The drawing under review shows one solid part. Ordinate dimensions are in mm from its lowest x, y, z. A direction names the side the tool comes from. Round coordinates to 2 decimals unless told otherwise and drop trailing zeros. Order: outer loops, then holes, each group sorted by start corner. A loop starts at its lowest first (then second) coordinate and runs counter-clockwise, first axis right, second up. Notation, with made-up numbers: (55.5, 55) -> (81.5, 55) arc R17 cw to (81.5, 71) -> close; hole circle Ø2 at (-36, 44). An arc over 180 degrees is marked (long way). Use a Markdown table: item, result. Add a question column.
1) Consider section B-B (y = 10). State the section outline as (x, z) points.
2) Wall thickness on line 1 along Y through (x, z) = (10, 23.85); line 2 along Y through (x, z) = (15.4, 10); line 3 along X through (y, z) = (13.5, 12.25): over which ranges is each line inside the solid? List them lowest first. Write a range as [from, to].
3) Clearance check with flat-ended pins moving along their axes: P1, Ø1.2, axis at x = 10, y = 5, coming from the -Z side; P2, Ø5, axis at x = 12.5, z = 6, coming from the -Y side; P3, Ø5, axis at x = 16, y = 17, coming from the -Z side; P4, Ø2.5, axis at x = 10.5, y = 6, coming from the -Z side. State where each tip first meets the part, or that it passes through.
4) Consider section C-C (z = 22). State the section outline as (x, y) points, plus the area to 3 significant figures.
5) Machinability: for the marked faces 4, 5 and 6, which of the approach directions +Z, -Z, +X, -X, +Y, -Y give a long, thin tool a straight path to every point of the face, cutting with its end or side? Answer none if there is none.
6) Draft analysis for pull direction X (two halves, no side actions). For the marked faces 1, 2 and 3, state which applies: pulls with the +X half, pulls with the -X half, needs draft (parallel to the pull), parting line crosses it, or undercut.
7) Consider section A-A (z = 17.75). State the section outline as (x, y) points, plus the area to 3 significant figures.
8) Consider section D-D (x = 10). State the section outline as (y, z) points, plus the area to 3 significant figures.
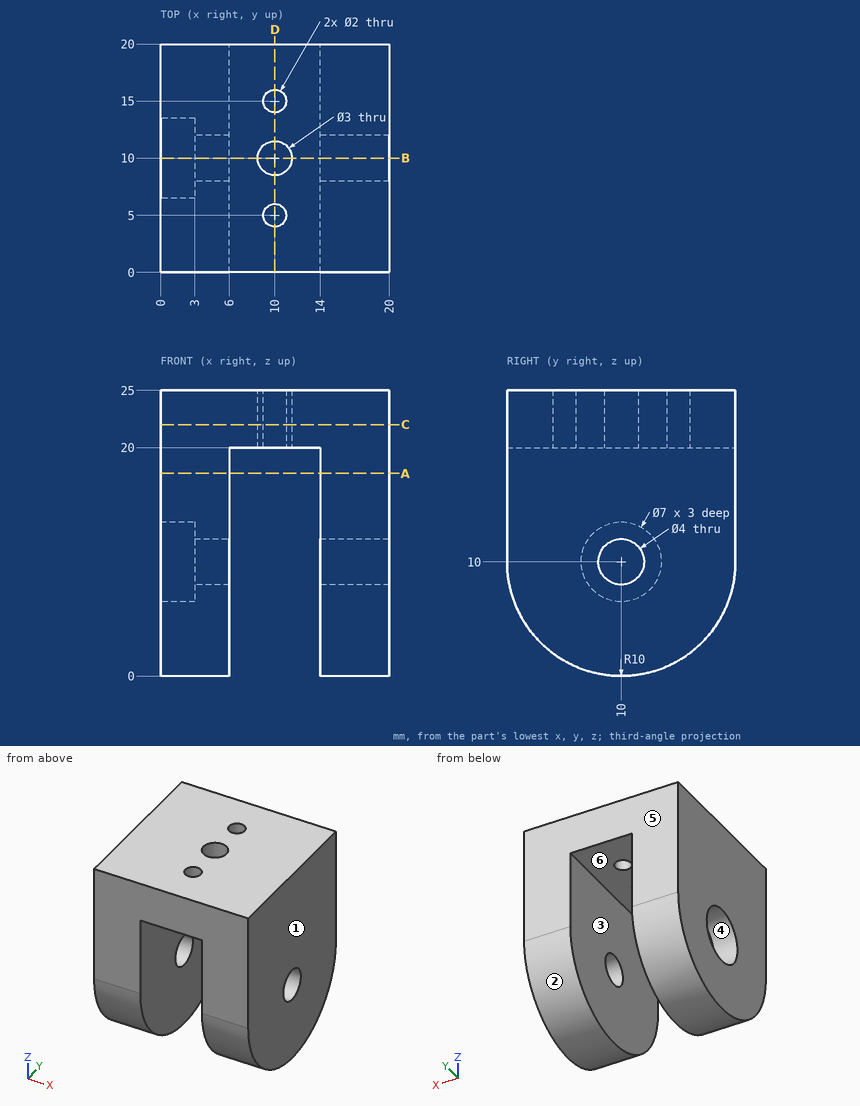
Results list:
| question | item | result |
|---|---|---|
| 1 | outline | (0, 0) -> (6, 0) -> (6, 8) -> (3, 8) -> (3, 6.5) -> (0, 6.5) -> close; (0, 13.5) -> (3, 13.5) -> (3, 12) -> (6, 12) -> (6, 20) -> (8.5, 20) -> (8.5, 25) -> (0, 25) -> close; (11.5, 20) -> (14, 20) -> (14, 12) -> (20, 12) -> (20, 25) -> (11.5, 25) -> close; (14, 0) -> (20, 0) -> (20, 8) -> (14, 8) -> close |
| 2 | line 1 | [0, 4], [6, 8.5], [11.5, 14], [16, 20] |
| 2 | line 2 | [0, 8], [12, 20] |
| 2 | line 3 | [0, 6], [14, 20] |
| 3 | P1 | through |
| 3 | P2 | y = 0.2 |
| 3 | P3 | z = 1.07 |
| 3 | P4 | z = 20 |
| 4 | outline | (0, 0) -> (20, 0) -> (20, 20) -> (0, 20) -> close; hole circle Ø3 at (10, 10); hole circle Ø2 at (10, 5); hole circle Ø2 at (10, 15) |
| 4 | area | 387 mm2 |
| 5 | face 4 | -X |
| 5 | face 5 | +Z, -Z, +X, -X, +Y |
| 5 | face 6 | -Z, +Y, -Y |
| 6 | face 1 | pulls with the +X half |
| 6 | face 2 | needs draft |
| 6 | face 3 | undercut |
| 7 | outline | (0, 0) -> (6, 0) -> (6, 20) -> (0, 20) -> close; (14, 0) -> (20, 0) -> (20, 20) -> (14, 20) -> close |
| 7 | area | 240 mm2 |
| 8 | outline | (0, 20) -> (4, 20) -> (4, 25) -> (0, 25) -> close; (6, 20) -> (8.5, 20) -> (8.5, 25) -> (6, 25) -> close; (11.5, 20) -> (14, 20) -> (14, 25) -> (11.5, 25) -> close; (16, 20) -> (20, 20) -> (20, 25) -> (16, 25) -> close |
| 8 | area | 65.0 mm2 |
